from build123d import *

# Parameters (mm, degrees)
SKETCH1_R            = 33.5
BOSS_EXTRUDE3_DEPTH  = 16.5
SKETCH2_W            = 20
SKETCH2_H            = 39
BOSS_EXTRUDE4_DEPTH  = 34.758
SKETCH3_R            = 10
SKETCH3_R_2          = 6.5
BOSS_EXTRUDE5_DEPTH  = 2
SKETCH3_3_R          = 6.5
BOSS_EXTRUDE6_DEPTH  = 3
SKETCH3_4_R          = 2.85
BOSS_EXTRUDE7_DEPTH  = 7.3
SKETCH5_W            = 11
SKETCH5_H            = 3.5
SKETCH5_W_2          = 3.5
SKETCH5_H_2          = 8
BOSS_EXTRUDE8_DEPTH  = 34.758
SKETCH6_W            = 11
SKETCH6_H            = 8
BOSS_EXTRUDE9_DEPTH  = 3.5
SKETCH7_R            = 2.5
BOSS_EXTRUDE10_DEPTH = 6
FILLET1_R            = 3.5
FILLET2_R            = 3.5
FILLET3_R            = 3.5
FILLET4_R            = 3.5
CUT_EXTRUDE11_DEPTH  = 3.5
CIRPATTERN4_COUNT    = 4
SKETCH14_3_R         = 1.25
CUT_EXTRUDE12_DEPTH  = 3.5
BOSS_EXTRUDE15_START = 60
SKETCH16_R           = 33.5
SKETCH16_R_2         = 30
BOSS_EXTRUDE15_DEPTH = 60
SKETCH17_W           = 60
SKETCH17_H           = 27
CUT_EXTRUDE13_DEPTH  = 33.5
SKETCH18_R           = 33.5
BOSS_EXTRUDE16_DEPTH = 3.5
CUT_EXTRUDE14_DEPTH  = 3.5
CIRPATTERN5_COUNT    = 4
CUT_EXTRUDE15_DEPTH  = 3.5


with BuildPart() as part:
    # Sketch1 → Boss-Extrude3 (new body)
    with BuildSketch(Plane.XY):
        Circle(SKETCH1_R)
    extrude(amount=BOSS_EXTRUDE3_DEPTH)

    # Sketch2 → Boss-Extrude4 (add)
    with BuildSketch(Plane.XY.offset(16.5)):
        Rectangle(SKETCH2_W, SKETCH2_H)
    extrude(amount=BOSS_EXTRUDE4_DEPTH)

    # Sketch3 → Boss-Extrude5 (add)
    with BuildSketch(Plane(origin=(0, 19.5, 0), x_dir=(1, 0, 0), z_dir=(0, 1, 0))):
        with Locations(Location((0, -41.258, 0), (0, 0, 270))):
            Circle(SKETCH3_R)
        with Locations(Location((0, -41.258, 0), (0, 0, 270))):
            Circle(SKETCH3_R_2, mode=Mode.SUBTRACT)
    extrude(amount=BOSS_EXTRUDE5_DEPTH)

    # Sketch3<3> → Boss-Extrude6 (add)
    with BuildSketch(Plane(origin=(0, 19.5, 0), x_dir=(1, 0, 0), z_dir=(0, 1, 0))):
        with Locations(Location((0, -41.258, 0), (0, 0, 270))):
            Circle(SKETCH3_3_R)
    extrude(amount=BOSS_EXTRUDE6_DEPTH)

    # Sketch3<4> → Boss-Extrude7 (add)
    with BuildSketch(Plane(origin=(0, 19.5, 0), x_dir=(1, 0, 0), z_dir=(0, 1, 0))):
        with Locations(Location((0, -41.258, 0), (0, 0, 270))):
            Circle(SKETCH3_4_R)
    extrude(amount=BOSS_EXTRUDE7_DEPTH)

    # Sketch5 → Boss-Extrude8 (add)
    with BuildSketch(Plane.XY.offset(51.258)):
        with Locations((0, -21.25)):
            Rectangle(SKETCH5_W, SKETCH5_H)
        with Locations((11.75, 7.5)):
            Rectangle(SKETCH5_W_2, SKETCH5_H_2)
        with Locations((-11.75, 7.5)):
            Rectangle(SKETCH5_W_2, SKETCH5_H_2)
    extrude(amount=-BOSS_EXTRUDE8_DEPTH)

    # Sketch6 → Boss-Extrude9 (add)
    with BuildSketch(Plane.XY.offset(51.258)):
        with Locations((0, 7.5)):
            Rectangle(SKETCH6_W, SKETCH6_H)
        Polygon((10, 11.5), (5.5, 11.5), (5.5, 3.5), (10, 3.5), (13.5, 3.5), (13.5, 11.5), align=None)
        Polygon((5.5, 3.5), (-5.5, 3.5), (-5.5, -19.5), (-5.5, -23), (5.5, -23), (5.5, -19.5), align=None)
        Polygon((-10, 11.5), (-13.5, 11.5), (-13.5, 3.5), (-10, 3.5), (-5.5, 3.5), (-5.5, 11.5), align=None)
    extrude(amount=BOSS_EXTRUDE9_DEPTH)

    # Sketch7 → Boss-Extrude10 (add)
    with BuildSketch(Plane.XZ.offset(23)):
        with Locations(Location((0, 41.258, 0), (0, 0, 270))):
            Circle(SKETCH7_R)
    extrude(amount=BOSS_EXTRUDE10_DEPTH)

    # Fillet1
    fillet1_edges = [part.edges().sort_by_distance(p)[0] for p in [
        (-13.5, 7.5, 54.758),
        (13.5, 7.5, 54.758),
    ]]
    fillet(fillet1_edges, radius=FILLET1_R)

    # Fillet2
    fillet2_edges = [part.edges().sort_by_distance(p)[0] for p in [
        (0, -23, 54.758),
    ]]
    fillet(fillet2_edges, radius=FILLET2_R)

    # Fillet3
    fillet3_edges = [part.edges().sort_by_distance(p)[0] for p in [
        (13.5, 7.5, 16.5),
    ]]
    fillet(fillet3_edges, radius=FILLET3_R)

    # Fillet4
    fillet4_edges = [part.edges().sort_by_distance(p)[0] for p in [
        (-13.5, 7.5, 16.5),
    ]]
    fillet(fillet4_edges, radius=FILLET4_R)

    # Sketch14 → Cut-Extrude11 (cut)
    with BuildSketch(Plane(origin=(0, 0, 0), x_dir=(-1, 0, 0), z_dir=(0, 0, -1))):
        with BuildLine():
            Line((0, 18), (0, 9))
            ThreePointArc((0, 9), (2.329371406, 8.693332437), (4.5, 7.794228634))
            Line((4.5, 7.794228634), (9, 15.588457268))
            ThreePointArc((9, 15.588457268), (4.658742812, 17.386664873), (0, 18))
        make_face()
        with BuildLine():
            ThreePointArc((-4.5, 7.794228634), (-2.329371406, 8.693332437), (0, 9))
            Line((0, 9), (0, 18))
            ThreePointArc((0, 18), (-4.658742812, 17.386664873), (-9, 15.588457268))
            Line((-9, 15.588457268), (-4.5, 7.794228634))
        make_face()
    cut_extrude11 = extrude(amount=-CUT_EXTRUDE11_DEPTH, mode=Mode.SUBTRACT)

    # CirPattern4: Cut-Extrude11 ×4 about axis
    cirpattern4_axis = Axis((0, 0, 0), (0, 0, 1))
    for i in range(1, CIRPATTERN4_COUNT):
        add(cut_extrude11.rotate(cirpattern4_axis, i * 360 / CIRPATTERN4_COUNT), mode=Mode.SUBTRACT)

    # Sketch14<3> → Cut-Extrude12 (cut)
    with BuildSketch(Plane(origin=(0, 0, 0), x_dir=(-1, 0, 0), z_dir=(0, 0, -1))):
        Circle(SKETCH14_3_R)
    extrude(amount=-CUT_EXTRUDE12_DEPTH, mode=Mode.SUBTRACT)

    # Sketch16 → Boss-Extrude15 (add)
    with BuildSketch(Plane(origin=(0, 0, 0), x_dir=(-1, 0, 0), z_dir=(0, 0, -1)).offset(BOSS_EXTRUDE15_START)):
        Circle(SKETCH16_R)
        Circle(SKETCH16_R_2, mode=Mode.SUBTRACT)
    extrude(amount=-BOSS_EXTRUDE15_DEPTH)

    # Sketch17 → Cut-Extrude13 (cut)
    with BuildSketch(Plane(origin=(0, 33.5, 0), x_dir=(1, 0, 0), z_dir=(0, 1, 0))):
        with Locations((0, 21.5)):
            Rectangle(SKETCH17_W, SKETCH17_H)
    extrude(amount=-CUT_EXTRUDE13_DEPTH, mode=Mode.SUBTRACT)

    # Sketch18 → Boss-Extrude16 (add)
    with BuildSketch(Plane(origin=(0, 0, -60), x_dir=(-1, 0, 0), z_dir=(0, 0, -1))):
        Circle(SKETCH18_R)
    extrude(amount=-BOSS_EXTRUDE16_DEPTH)

    # Sketch18<3> → Cut-Extrude14 (cut)
    with BuildSketch(Plane(origin=(0, 0, -60), x_dir=(-1, 0, 0), z_dir=(0, 0, -1))):
        with BuildLine():
            ThreePointArc((-4.5, 7.794228634), (-2.329371406, 8.693332437), (0, 9))
            Line((0, 9), (0, 18))
            ThreePointArc((0, 18), (-4.658742812, 17.386664873), (-9, 15.588457268))
            Line((-9, 15.588457268), (-4.5, 7.794228634))
        make_face()
        with BuildLine():
            Line((0, 18), (0, 9))
            ThreePointArc((0, 9), (2.329371406, 8.693332437), (4.5, 7.794228634))
            Line((4.5, 7.794228634), (9, 15.588457268))
            ThreePointArc((9, 15.588457268), (4.658742812, 17.386664873), (0, 18))
        make_face()
    cut_extrude14 = extrude(amount=-CUT_EXTRUDE14_DEPTH, mode=Mode.SUBTRACT)

    # CirPattern5: Cut-Extrude14 ×4 about axis
    cirpattern5_axis = Axis((0, 0, 16.5), (0, 0, -1))
    for i in range(1, CIRPATTERN5_COUNT):
        add(cut_extrude14.rotate(cirpattern5_axis, i * 360 / CIRPATTERN5_COUNT), mode=Mode.SUBTRACT)

    # Sketch18<4> → Cut-Extrude15 (cut)
    with BuildSketch(Plane(origin=(0, 0, -60), x_dir=(-1, 0, 0), z_dir=(0, 0, -1))):
        with BuildLine():
            Line((0, 1.75), (0, 0))
            Line((0, 0), (0.875, 1.515544457))
            ThreePointArc((0.875, 1.515544457), (0.452933329, 1.690370196), (0, 1.75))
        make_face()
        with BuildLine():
            Line((-0.875, 1.515544457), (0, 0))
            Line((0, 0), (0, 1.75))
            ThreePointArc((0, 1.75), (-0.452933329, 1.690370196), (-0.875, 1.515544457))
        make_face()
        with BuildLine():
            Line((0.875, 1.515544457), (0, 0))
            Line((0, 0), (-0.875, 1.515544457))
            ThreePointArc((-0.875, 1.515544457), (-0.875, -1.515544457), (1.75, 0))
            ThreePointArc((1.75, 0), (1.515544457, 0.875), (0.875, 1.515544457))
        make_face()
    extrude(amount=-CUT_EXTRUDE15_DEPTH, mode=Mode.SUBTRACT)


solid = part.part
Check sheet for the modelled part. Datum: model origin and axes. Units: mm. A direction names the side the tool comes from. Give positions to 0.01 mm unless a question says otherwise; leave off trailing zeros. Write each loop counter-clockwise with the first axis right and the second up, starting at its lowest first coordinate (ties: lowest second). Pieces come first, ordered by that corner, then holes. Notation, with made-up numbers: (67.5, -15.5) -> (111.5, -15.5) arc R28 ccw to (111.5, 14.5) -> close; hole circle Ø5 at (35, 77.25). An arc over 180 degrees is marked (long way). One line per item, written item: value. Start each with the question number.
Item 1: Gauge pin test, flat ends, axial feed: pin 1 (12 mm diameter, centred on x = -12.5, z = 32.5, fed in from +Y); pin 2 (1.3 mm diameter, centred on x = -8, z = 28.5, fed in from -Y); pin 3 (6 mm diameter, centred on y = -14, z = -45, fed in from -X). Record the tip position at first contact, or that the pin passes through.
Item 2: Material ranges on probe 1 along Z at (x, y) = (16.5, -25); probe 2 along X at (y, z) = (0, -39), recorded low to high. Write a range as from..to.
Item 3: Section check C-C on z = -37. Record the cut outline in (x, y), then the cut area to 3 significant figures.
Item 4: Section check D-D on x = 27. Record the cut outline in (y, z), then the cut area to 3 significant figures.
Item 5: Section check A-A on x = -12. Record the cut outline in (y, z), then the cut area to 3 significant figures.
Item 6: Section check B-B on x = -20. Record the cut outline in (y, z).
Item 7: Tool access check on faces 1 (the cylindrical face through (0.44, 20.486, 31.268)), 2 (the flat face through (-8, -8, 51.258)), 3 (the flat face through (0, -6, -56.5)), 4 (the flat face through (0, -29, 41)), 5 (the flat face through (-6.782, -11.746, 1.726)). Record the directions out of +Z, -Z, +X, -X, +Y, -Y that give a thin tool (end or side, any length) a straight path to the whole face; none if there is none.
Item 8: Draft check along Y on faces 6 (the flat face through (-5.5, -20, 40)), 7 (the flat face through (-11.746, 6.782, 1.726)), 8 (the flat face through (0, 19.5, 26)). Enter one of: +Y half, -Y half, draft (parallel to the pull), parting line (faces both ways), or undercut.
Results list:
1. pin 1: y = 21.5
1. pin 2: y = -19.5
1. pin 3: x = -31.64
2. probe 1: -60..-56.5, 0..16.5
2. probe 2: -33.5..-30, 30..33.5
3. outline: circle Ø67 at (0, 0); hole circle Ø60 at (0, 0)
3. area: 698 mm²
4. outline: (-19.83, -60) -> (19.83, -60) -> (19.83, -35) -> (13.08, -35) -> (13.08, -56.5) -> (-13.08, -56.5) -> (-13.08, 0) -> (13.08, 0) -> (13.08, -8) -> (19.83, -8) -> (19.83, 16.5) -> (-19.83, 16.5) -> close
4. area: 1,370 mm²
5. outline: (-31.28, -60) -> (-6.93, -60) -> (-6.93, -56.5) -> (-27.5, -56.5) -> (-27.5, 0) -> (-6.93, 0) -> (-6.93, 3.5) -> (6.93, 3.5) -> (6.93, 0) -> (27.5, 0) -> (27.5, -8) -> (31.28, -8) -> (31.28, 16.5) -> (11.5, 16.5) -> (11.5, 54.13) -> (3.5, 54.13) -> (3.5, 16.5) -> (-31.28, 16.5) -> close; (6.93, -60) -> (31.28, -60) -> (31.28, -35) -> (27.5, -35) -> (27.5, -56.5) -> (6.93, -56.5) -> close
5. area: 1,780 mm²
6. outline: (-26.87, -60) -> (26.87, -60) -> (26.87, -35) -> (22.36, -35) -> (22.36, -56.5) -> (-22.36, -56.5) -> (-22.36, 0) -> (22.36, 0) -> (22.36, -8) -> (26.87, -8) -> (26.87, 16.5) -> (-26.87, 16.5) -> close
7. face 1: +Y
7. face 2: +Z, -X, -Y
7. face 3: none
7. face 4: +Z, +X, -X, -Y
7. face 5: -Z
8. face 6: draft
8. face 7: undercut
8. face 8: +Y half
